Autodesk Fusion 360 part; units mm, degrees
sketch "Sketch1" plane through (0, 0, 0) normal (0, 0, 1) x (1, 0, 0)
  line L0 (0, 0) -> (30, 0)
  line L1 (30, 0) -> (30, 50)
  line L2 (30, 50) -> (0, 50)
  line L3 (0, 50) -> (0, 0)
  dimension "d1" = 30
  dimension "d2" = 50
extrude "Extrude1" add sketch "Sketch1" along normal blind 5
sketch "Sketch2" plane through (0, 0, 5) normal (0, 0, 1) x (-1, 0, 0)
  line L0 (0, -50) -> (0, 0)
  line L1 (0, 0) -> (-30, 0)
  line L2 (-30, 0) -> (-30, -50)
  line L3 (-30, -50) -> (0, -50)
  line L4 (0, -50) -> (-5, -50)
  line L5 (-5, -50) -> (-5, 0)
  line L6 (-5, 0) -> (0, 0)
  line L7 (0, 0) -> (0, -50)
extrude "Extrude2" add sketch "Sketch2" along normal blind 20 contours L0 L1 L3 L4 L5 L6 L7
sketch "Sketch3" plane through (0, 0, 5) normal (0, 0, 1) x (-1, 0, 0)
  line L0 (-5, -50) -> (-5, 0)
  line L1 (-5, 0) -> (-30, 0)
  line L2 (-30, 0) -> (-30, -50)
  line L3 (-30, -50) -> (-5, -50)
  line L4 (-30, 0) -> (-23, 0)
  line L5 (-23, 0) -> (-23, -7)
  line L6 (-23, -7) -> (-30, -7)
  line L7 (-30, -7) -> (-30, 0)
  line L8 (-30, -50) -> (-23, -50)
  line L9 (-23, -50) -> (-23, -43)
  line L10 (-23, -43) -> (-30, -43)
  line L11 (-30, -43) -> (-30, -50)
  line L12 (-5, -50) -> (-12, -50)
  line L13 (-12, -50) -> (-12, -43)
  line L14 (-12, -43) -> (-5, -43)
  line L15 (-5, -43) -> (-5, -50)
  line L16 (-5, 0) -> (-12, 0)
  line L17 (-12, 0) -> (-12, -7)
  line L18 (-12, -7) -> (-5, -7)
  line L19 (-5, -7) -> (-5, 0)
  circle A0 centre (-18, -12.5) radius 8
  circle A1 centre (-18, -37.5) radius 8
  dimension "d7" = 7
  dimension "d8" = 7
  dimension "d9" = 7
  dimension "d10" = 7
  dimension "d11" = 7
  dimension "d12" = 7
  dimension "d13" = 7
  dimension "d14" = 7
  dimension "d16" = 16
  dimension "d17" = 16
extrude "Extrude3" cut sketch "Sketch3" against normal blind 5 contours L9 L10 A1 | L5 L6 A0 picked at (-16.0576, -35.427) picked at (-16.0576, -14.573)
extrude "Extrude4" add sketch "Sketch3" along normal blind 5 contours L0 L3 L12 L13 L14 L15 | L0 L1 L16 L17 L18 L19 | L2 L3 L8 L9 L10 L11 A1 | L1 L2 L4 L5 L6 L7 A0
extrude "Extrude5" cut sketch "Sketch3" against normal blind 5 contours L9 L10 A1 | L5 L6 A0 picked at (-16.0576, -35.427) picked at (-16.0576, -14.573)
chamfer "Chamfer1" distance 1 angle 45 2 edges at (12, 7, 7.5) (12, 43, 7.5)
sketch "Sketch4" plane through (30, 0, 0) normal (1, 0, 0) x (0, 1, 0)
  line L0 (0, 0) -> (50, 0)
  line L1 (50, 0) -> (50, 10)
  line L2 (50, 10) -> (43, 10)
  line L3 (43, 10) -> (43, 5)
  line L4 (43, 5) -> (7, 5)
  line L5 (7, 5) -> (7, 10)
  line L6 (7, 10) -> (0, 10)
  line L7 (0, 10) -> (0, 0)
  line L8 (20.5, 5.0863) -> (4.5107, 5.0863)
  line L9 (4.5107, 5.0863) -> (4.5107, 0)
  line L10 (4.5107, 0) -> (20.5, 0)
  line L11 (20.5, 0) -> (20.5, 5.0863)
  line L12 (29.4867, 0) -> (45.5, 0)
  line L13 (45.5, 0) -> (45.5, 5.0968)
  line L14 (45.5, 5.0968) -> (29.4867, 5.0968)
  line L15 (29.4867, 5.0968) -> (29.4867, 0)
  line L16 (7, 10) -> (4.5107, 10)
  line L17 (4.5107, 10) -> (4.5107, 5.0863)
  line L18 (4.5107, 5.0863) -> (7, 5.0863)
  line L19 (7, 5.0863) -> (7, 10)
  line L20 (43, 10) -> (45.5, 10)
  line L21 (45.5, 10) -> (45.5, 5.0968)
  line L22 (45.5, 5.0968) -> (43, 5.0968)
  line L23 (43, 5.0968) -> (43, 10)
extrude "Extrude6" cut sketch "Sketch4" against normal blind 12 contours L0 L4 L5 L8 L9 L10 L11 L18 | L5 L6 L8 L16 L17 L18 L19 | L0 L3 L4 L12 L13 L14 L15 L22 | L2 L3 L14 L20 L21 L22 L23
sketch "Sketch5" plane through (0, 0, 0) normal (-1, 0, 0) x (0, -1, 0)
  line L0 (-50, 0) -> (0, 0)
  line L1 (0, 0) -> (0, 25)
  line L2 (0, 25) -> (-50, 25)
  line L3 (-50, 25) -> (-50, 0)
  circle A0 centre (-25, 17) radius 2.45
  circle A1 centre (-38.5, 17) radius 1
  circle A2 centre (-11.5, 17) radius 1
  dimension "d27" = 4.9
  dimension "d36" = 2
  dimension "d37" = 2
extrude "Extrude7" cut sketch "Sketch5" against normal blind 5 contours A0 | A1 | A2
sketch "Sketch6" plane through (5, 0, 0) normal (1, 0, 0) x (0, 1, 0)
  circle A0 centre (25, 17) radius 2.45
  line L0 (0, 10) -> (7, 10)
  line L1 (7, 10) -> (7, 5)
  line L2 (7, 5) -> (43, 5)
  line L3 (43, 5) -> (43, 10)
  line L4 (43, 10) -> (50, 10)
  line L5 (50, 10) -> (50, 25)
  line L6 (50, 25) -> (0, 25)
  line L7 (0, 25) -> (0, 10)
  line L8 (0, 12) -> (9, 12)
  line L9 (9, 12) -> (9, 14)
  line L10 (9, 14) -> (0, 14)
  line L11 (0, 14) -> (0, 12)
  line L12 (50, 12) -> (41, 12)
  line L13 (41, 12) -> (41, 14)
  line L14 (41, 14) -> (50, 14)
  line L15 (50, 14) -> (50, 12)
  circle A1 centre (11.5, 17) radius 1
  circle A2 centre (38.5, 17) radius 1
extrude "Extrude8" add sketch "Sketch6" along normal blind 7 contours L7 L8 L9 L10 L11 | L5 L12 L13 L14 L15
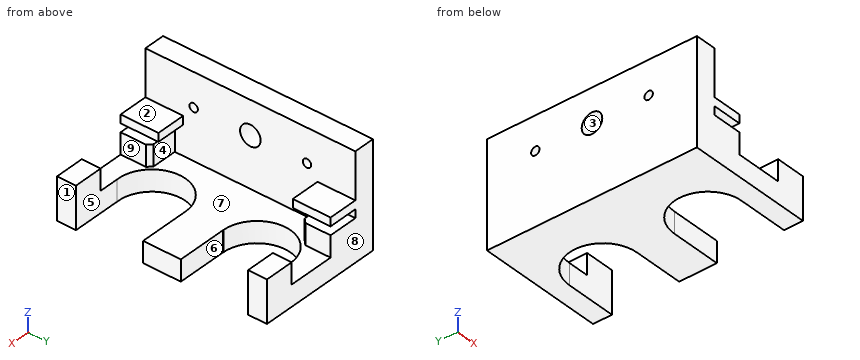
Check sheet for the modelled part. Datum: model origin and axes. Units: mm. Face numbers are marked on the shaded views. A direction names the side the tool comes from. Round coordinates to 2 decimals unless told otherwise and drop trailing zeros. Loops run counter-clockwise (first coordinate to the right, second up) from the corner with the lowest first, then second, coordinate; pieces in that order, holes last.
1. Mould release check, pull along Y, two halves, no side actions. Record for the marked faces 6, 7, 8 and 9: released by +Y, released by -Y, zero draft, split by the parting line, or undercut.
2. Sectioned sample at A-A on x = 20.25. Record the boundary of the cut face in (y, z), and give its area (3 significant figures).
3. Scan lines: probe 1 along Y at (x, z) = (22.5, 4.5); probe 2 along Z at (x, y) = (3.6, 11.5); probe 3 along Z at (x, y) = (5.25, 8). Record each from-to range of solid material in increasing order.
4. Sectioned sample at D-D on y = 46.5. Record the boundary of the cut face in (x, z).
5. Sectioned sample at C-C on z = 17. Record the boundary of the cut face in (x, y), and give its area (4 significant figures).
6. Sectioned sample at B-B on y = 25. Record the boundary of the cut face in (x, z), and give its area (4 significant figures).
7. Gauge pin test, flat ends, axial feed: pin 1 Ø2 at (x, y) = (7.5, 4) entering from +Z; pin 2 Ø3.5 at (x, y) = (28, 48) entering from +Z; pin 3 Ø8 at (x, z) = (20, 14.5) entering from -Y; pin 4 Ø1 at (y, z) = (42.5, 21) entering from +X. Record the tip position at first contact, or that the pin passes through.
8. Set-up check for the marked faces 1, 2, 3, 4 and 5: record each of +Z, -Z, +X, -X, +Y, -Y from which the full face is reachable in a straight line by a thin tool's end or side.
Recorded:
1. face 6: undercut
1. face 7: undercut
1. face 8: released by +Y
1. face 9: zero draft
2. outline: (0, 0) - (4.51, 0) - (4.51, 5) - (0, 5) - close; (20.5, 0) - (29.49, 0) - (29.49, 5) - (20.5, 5) - close; (45.5, 0) - (50, 0) - (50, 5) - (45.5, 5) - close
2. area: 90.0 mm2
3. probe 1: y = 0 to 4.51, 20.5 to 29.49, 45.5 to 50
3. probe 2: z = 0 to 16, 18 to 25
3. probe 3: z = 0 to 5, 12 to 14
4. outline: (0, 0) - (30, 0) - (30, 10) - (23, 10) - (23, 5) - (12, 5) - (12, 10) - (5, 10) - (5, 12) - (12, 12) - (12, 14) - (5, 14) - (5, 25) - (0, 25) - close
5. outline: (0, 0) - (5, 0) - (5, 10.5) - (0, 10.5) - close; (0, 12.5) - (5, 12.5) - (5, 22.55) - (0, 22.55) - close; (0, 27.45) - (5, 27.45) - (5, 37.5) - (0, 37.5) - close; (0, 39.5) - (5, 39.5) - (5, 50) - (0, 50) - close
5. area: 205.5 mm2
6. outline: (0, 0) - (30, 0) - (30, 5) - (5, 5) - (5, 14.55) - (0, 14.55) - close; (0, 19.45) - (5, 19.45) - (5, 25) - (0, 25) - close
6. area: 225.5 mm2
7. pin 1: stops at z = 14
7. pin 2: stops at z = 10
7. pin 3: passes through
7. pin 4: stops at x = 5
8. face 1: +Z, -Z, +X, +Y, -Y
8. face 2: +Z, +X, +Y, -Y
8. face 3: +X, -X
8. face 4: +X
8. face 5: +Z, -Z, +X
